The model under review builds one solid part; all positions refer to its coordinate system, in mm. Face numbers are marked on the shaded views. Coordinates: 2 decimals unless noted, no trailing zeros. Put each result on its own line as item: value. Start each with the question number.
Item 1: To check wall thickness, follow L1, parallel to Z at x = 34.5, y = 14.25; L2, parallel to X at y = 14, z = 8; L3, parallel to X at y = 20, z = 3.25. State the ranges of each line that lie inside material, in increasing order. Write a range as [from, to].
Item 2: For pin 1 (1.6 mm diameter, centred on x = 35, y = 13.5, fed in from +Z); pin 2 (3 mm diameter, centred on y = 14, z = 8, fed in from +X); pin 3 (1.1 mm diameter, centred on x = 33.5, y = 14, fed in from -Z), all flat-tipped, find the tip position at first contact; note any pin that passes through.
Item 3: Mouldability with a two-part tool opening along Y and no side actions: class the marked faces 1 and 2 as pulls with the +Y half, pulls with the -Y half, needs draft (parallel to the pull), parting line crosses it, or undercut.
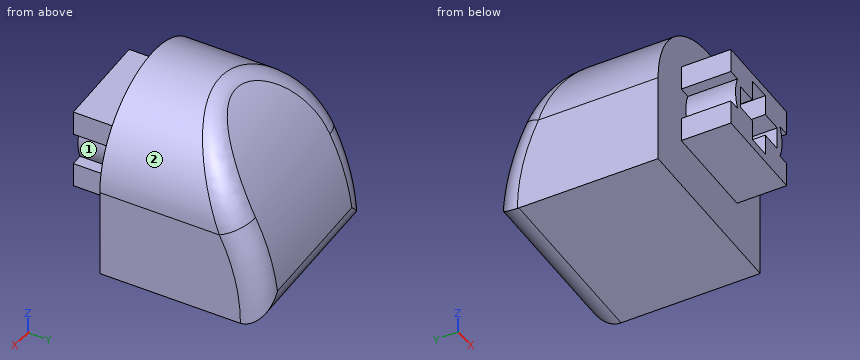
```python
from build123d import *

# Parameters (mm, degrees)
PAD112_DEPTH               = 3
PAD126_DEPTH               = 10
POCKET064_DEPTH            = 5.5
FILLET009_R                = 1.5
BODY181005_ROLL_ANGLE      = 89.997092
BODY181005_PITCH_ANGLE     = 5.8e-05
BODY181005_PLACEMENT_ANGLE = -177.708532


with BuildPart() as part:
    # Sketch208 → Pad112 (new body)
    with BuildSketch(Plane.XY):
        with BuildLine():
            ThreePointArc((-2.291288, 1), (-2.5, 0), (-2.291288, -1))
            Line((-3, -1), (-2.291288, -1))
            Line((-3, -2.5), (-3, -1))
            Line((-3, -2.5), (3, -2.5))
            Line((3, -2.5), (3, -1))
            Line((3, -1), (2.291288, -1))
            ThreePointArc((2.291288, -1), (2.5, 0), (2.291288, 1))
            Line((3, 1), (2.291288, 1))
            Line((3, 2.5), (3, 1))
            Line((-3, 2.5), (3, 2.5))
            Line((-3, 2.5), (-3, 1))
            Line((-3, 1), (-2.291288, 1))
        make_face()
        Polygon((-1.979899, 0.7), (-0.7, 0.7), (-0.7, 1.979899), (0.7, 1.979899), (0.7, 0.7), (1.979899, 0.7), (1.979899, -0.7), (0.7, -0.7), (0.7, -1.979899), (-0.7, -1.979899), (-0.7, -0.7), (-1.979899, -0.7), align=None, mode=Mode.SUBTRACT)
    extrude(amount=PAD112_DEPTH)


with BuildPart() as part_1:
    # Body167 placement: moved
    add(part.part.moved(Location((0, 0, 6))))

    # Sketch240 → Pad126 (new body)
    with BuildSketch(Plane.XY.offset(9)):
        with BuildLine():
            Line((5.5, 0), (5.5, -5.5))
            Line((5.5, -5.5), (-5.5, -5.5))
            Line((-5.5, -5.5), (-5.5, 0))
            ThreePointArc((5.5, 0), (0, 5.5), (-5.5, 0))
        make_face()
    extrude(amount=PAD126_DEPTH)

    # Sketch241 → Pocket064 (cut, symmetric)
    with BuildSketch(Plane(origin=(0, -5.5, 5), x_dir=(0, 1, 0), z_dir=(1, 0, 0))):
        with BuildLine():
            ThreePointArc((14, 0), (9.899495, 9.899495), (0, 14))
            Line((0, 14), (14, 14))
            Line((14, 14), (14, 0))
        make_face()
    extrude(amount=POCKET064_DEPTH, both=True, mode=Mode.SUBTRACT)

    # Fillet009
    fillet009_edges = [part_1.edges().sort_by_distance(p)[0] for p in [
        (5.5, -2.693, 18.715712),
        (0, 5.5, 13.660254),
        (-5.5, -2.693, 18.715712),
        (0, -5.5, 19),
    ]]
    fillet(fillet009_edges, radius=FILLET009_R)


with BuildPart() as part_2:
    # Body181005 roll: moved
    add(part_1.part.rotate(Axis((0, 0, 0), (1, 0, 0)), BODY181005_ROLL_ANGLE))


with BuildPart() as part_3:
    # Body181005 pitch: moved
    add(part_2.part.rotate(Axis((0, 0, 0), (0, 1, 0)), BODY181005_PITCH_ANGLE))


with BuildPart() as part_4:
    # Body181005 placement: moved
    add(part_3.part.moved(Location((34.990016, 5.999193, 8.017979))).rotate(Axis((34.990016, 5.999193, 8.017979), (0, 0, 1)), BODY181005_PLACEMENT_ANGLE))


solid = part_4.part
```
Report:
1. L1: [5.52, 6.04], [10, 10.52]
1. L2: [32.17, 32.69], [36.65, 37.17]
1. L3: [28.93, 39.93]
2. pin 1: z = 10.52
2. pin 2: x = 40.13
2. pin 3: z = 5.52
3. face 1: undercut
3. face 2: parting line crosses it
